Can you work these out from the model? Positions are in its coordinate system, mm. A direction names the side the tool comes from. Round coordinates to 2 decimals unless told otherwise and drop trailing zeros. Order: outer loops, then holes, each group sorted by start corner. A loop starts at its lowest first (then second) coordinate and runs counter-clockwise, first axis right, second up. Notation, with made-up numbers: (-36.5, 39) -> (-18.5, 39) arc R18 cw to (-18.5, 62) -> close; hole circle Ø6 at (-27, -15.5). An arc over 180 degrees is marked (long way). One line per item, written item: value.
Autodesk Inventor part; units mm, degrees
ref_plane "YZ Plane" through (0, 0, 0) normal (1, 0, 0) x (0, 1, 0)
ref_plane "XZ Plane" through (0, 0, 0) normal (0, 1, 0) x (-1, 0, 0)
ref_plane "XY Plane" through (0, 0, 0) normal (0, 0, 1) x (1, 0, 0)
sketch "Sketch2" plane through (0, 0, 0) normal (0, 0, 1) x (1, 0, 0)
  line L0 (0, 0) -> (0, 30)
  line L1 (0, 30) -> (-16.5, 30)
  line L2 (0, 0) -> (-13, 0)
  line L3 (-13, 0) -> (-16.5, 0)
  line L4 (-13, 30) -> (-13, 20)
  line L5 (-13, 20) -> (-14.35, 20)
  line L6 (-14.35, 20) -> (-14.35, 17.2)
  line L7 (-14.35, 17.2) -> (-13, 17.2)
  line L8 (-13, 17.2) -> (-13, 0)
  line L9 (-16.5, 13) -> (-15.8, 13)
  line L10 (-15.8, 13) -> (-15.8, 10.5)
  line L11 (-15.8, 10.5) -> (-16.5, 10.5)
  line L12 (-16.5, 30) -> (-16.5, 15)
  line L13 (-16.5, 15) -> (-18, 15)
  line L14 (-18, 15) -> (-18, 13)
  line L15 (-18, 13) -> (-16.5, 13)
  line L16 (-16.5, 10.5) -> (-16.5, 1.5)
  line L17 (-16.5, 1.5) -> (-13, 1.5)
  dimension "d4" = 30
  dimension "d5" = 16.5
  dimension "d6" = 13
  dimension "d7" = 10
  dimension "d8" = 1.35
  dimension "d9" = 2.8
  dimension "d13" = 17
  dimension "d14" = 0.7
  dimension "d15" = 2.5
  dimension "d18" = 15
  dimension "d19" = 1.5
  dimension "d20" = 10.5
  dimension "d21" = 9
revolve "Revolution1" add sketch "Sketch2" angle 360 about axis through (0, 0, 0) along (0, 1, 0) contours L4 L5 L6 L7 L8 L17 L16 L11 L10 L9 L15 L14 L13 L12 L1
thread "Thread3"
properties part number "Heated tube-top connector" material "Polypropylene"
Q1. Will these pins go through, and if not, where does the flat tip stop? pin 1 Ø1.5 at (y, z) = (10, 2.5) entering from +X; pin 2 Ø1 at (x, y) = (-1, 15) entering from -Z; pin 3 Ø3 at (x, y) = (11, 25) entering from -Z.
Answers below:
pin 1: x = 16.41
pin 2: z = -17.99
pin 3: z = -13.49
Q2. Please list where these lines run through material, in increasing order: line 1 along Z through (x, y) = (0, 18.25); line 2 along Y through (x, z) = (-4, 13); line 3 along Y through (x, z) = (-5.5, 15).
Answers below:
line 1: -16.5 to -14.35, 14.35 to 16.5
line 2: 1.5 to 17.2, 20 to 30
line 3: 1.5 to 10.5, 13 to 30
Q3. On a 3-axis mill with a long thin cutter (end or side, diameter ignored), from which of +Z, -Z, +X, -X, +Y, -Y can I reach the whole of each face in a straight line? I mean faces 1 (the face through (0.1, 30, -13.4)), 2 (the face through (-16, 10.5, 0)), 3 (the face through (-15.24, 22.4, 6.32)), 4 (the face through (-15.24, 5.94, 6.32)). Say none if no direction works.
Answers below:
face 1: +Z, -Z, +X, -X, +Y
face 2: none
face 3: +Y
face 4: -Y
Q4. I want a section at B-B on z = 0. List the corners of the cut face in (x, y) for me.
Answers below:
outline: (-18, 13) -> (-15.8, 13) -> (-15.8, 10.5) -> (-16.5, 10.5) -> (-16.5, 1.5) -> (-13, 1.5) -> (-13, 17.2) -> (-14.35, 17.2) -> (-14.35, 20) -> (-13, 20) -> (-13, 30) -> (-16.5, 30) -> (-16.5, 15) -> (-18, 15) -> close; (13, 1.5) -> (16.5, 1.5) -> (16.5, 10.5) -> (15.8, 10.5) -> (15.8, 13) -> (18, 13) -> (18, 15) -> (16.5, 15) -> (16.5, 30) -> (13, 30) -> (13, 20) -> (14.35, 20) -> (14.35, 17.2) -> (13, 17.2) -> close
Q5. We'd pull the mould along X, two halves only. Please class faces 5 (the face through (2.343, 13.986, -17.847)), 6 (the face through (0, 13, -16)), 7 (the face through (13, 17.2, 2)): released by +X, released by -X, zero draft, split by the parting line, or undercut.
Answers below:
face 5: split by the parting line
face 6: zero draft
face 7: undercut
Q6. I want a section at C-C on y = 9.5. List the corners of the cut face in (x, z) for me, plus the area to 3 significant figures.
Answers below:
outline: circle Ø33 at (0, 0); hole circle Ø26 at (0, 0)
area: 324 mm^2
Q7. I want a section at A-A on x = 0. List the corners of the cut face in (y, z) for me.
Answers below:
outline: (1.5, -16.5) -> (10.5, -16.5) -> (10.5, -15.8) -> (13, -15.8) -> (13, -18) -> (15, -18) -> (15, -16.5) -> (30, -16.5) -> (30, -13) -> (20, -13) -> (20, -14.35) -> (17.2, -14.35) -> (17.2, -13) -> (1.5, -13) -> close; (1.5, 13) -> (17.2, 13) -> (17.2, 14.35) -> (20, 14.35) -> (20, 13) -> (30, 13) -> (30, 16.5) -> (15, 16.5) -> (15, 18) -> (13, 18) -> (13, 15.8) -> (10.5, 15.8) -> (10.5, 16.5) -> (1.5, 16.5) -> close
